Check sheet for the modelled part. Datum: model origin and axes. Units: mm. A direction names the side the tool comes from. Round coordinates to 2 decimals unless told otherwise and drop trailing zeros. Write each loop counter-clockwise with the first axis right and the second up, starting at its lowest first coordinate (ties: lowest second). Pieces come first, ordered by that corner, then holes. Notation, with made-up numbers: M -16,40.5 L -3,40.5 A19 ccw -3,50.5 Z; hole C 61,-30 d5. An arc over 180 degrees is marked long. Answer in a Markdown table with one row per item.
```python
from build123d import *

# Parameters (mm, degrees)
SKETCH1_W           = 550
SKETCH1_H           = 105
SKETCH1_R           = 50
BOSS_EXTRUDE2_DEPTH = 80
FILLET4_R           = 50
FILLET5_R           = 50
SKETCH11_W          = 150
SKETCH11_H          = 104.268109322
BOSS_EXTRUDE3_DEPTH = 80
SKETCH12_R          = 5
BOSS_EXTRUDE4_DEPTH = 120
FILLET8_R           = 50
FILLET9_R           = 50
FILLET10_R          = 50
SKETCH13_R          = 16.1
CUT_EXTRUDE1_DEPTH  = 150


with BuildPart() as part:
    # Sketch1 → Boss-Extrude2 (new body)
    with BuildSketch(Plane(origin=(0, 0, 0), x_dir=(1, 0, 0), z_dir=(0, 1, 0))):
        Rectangle(SKETCH1_W, SKETCH1_H)
        with Locations((-220, 0)):
            Circle(SKETCH1_R, mode=Mode.SUBTRACT)
        with Locations((125, 0)):
            Circle(SKETCH1_R, mode=Mode.SUBTRACT)
    extrude(amount=BOSS_EXTRUDE2_DEPTH)

    # Fillet4
    fillet4_edges = [part.edges().sort_by_distance(p)[0] for p in [
        (275, 40, 52.5),
    ]]
    fillet(fillet4_edges, radius=FILLET4_R)

    # Fillet5
    fillet5_edges = [part.edges().sort_by_distance(p)[0] for p in [
        (275, 40, -52.5),
    ]]
    fillet(fillet5_edges, radius=FILLET5_R)

    # Sketch11 → Boss-Extrude3 (add)
    with BuildSketch(Plane(origin=(0, 80, 0), x_dir=(1, 0, 0), z_dir=(0, 1, 0))):
        with Locations((-200, 0.365945339)):
            Rectangle(SKETCH11_W, SKETCH11_H)
    extrude(amount=BOSS_EXTRUDE3_DEPTH)

    # Sketch12 → Boss-Extrude4 (add)
    with BuildSketch(Plane.XZ.offset(-80)):
        with Locations((-220, 0)):
            Circle(SKETCH12_R)
    extrude(amount=BOSS_EXTRUDE4_DEPTH)

    # Fillet8
    fillet8_edges = [part.edges().sort_by_distance(p)[0] for p in [
        (-275, 40, 52.5),
    ]]
    fillet(fillet8_edges, radius=FILLET8_R)

    # Fillet9
    fillet9_edges = [part.edges().sort_by_distance(p)[0] for p in [
        (-275, 80, -52.5),
    ]]
    fillet(fillet9_edges, radius=FILLET9_R)

    # Fillet10
    fillet10_edges = [part.edges().sort_by_distance(p)[0] for p in [
        (-125, 160, -0.365945339),
    ]]
    fillet(fillet10_edges, radius=FILLET10_R)

    # Sketch13 → Cut-Extrude1 (cut)
    with BuildSketch(Plane(origin=(275, 0, 0), x_dir=(0, 0, -1), z_dir=(1, 0, 0))):
        with Locations((0, 23.9)):
            Circle(SKETCH13_R)
    extrude(amount=-CUT_EXTRUDE1_DEPTH, mode=Mode.SUBTRACT)


solid = part.part
```
1. Draft check along X on faces 1 (the face through (85, 39, 30)), 2 (the face through (-215.23, 20.84, 1.5)), 3 (the face through (-260.742, 78.88, -37.464)), 4 (the face through (-180, 119, 51.768)). Enter one of: +X half, -X half, draft (parallel to the pull), parting line (faces both ways), or undercut.
Found:
| item | result |
|---|---|
| face 1 | undercut |
| face 2 | undercut |
| face 3 | -X half |
| face 4 | draft |
2. Scan lines: L1, parallel to Y at x = 211, z = 0; L2, parallel to Z at x = 125, y = 33; L3, parallel to Z at x = -220, y = 23. Record each from-to range of solid material in increasing order.
Found:
| item | result |
|---|---|
| L1 | y = 0 to 7.8, 40 to 80 |
| L2 | z = -52.5 to -50, 50 to 52.5 |
| L3 | z = -52.5 to -50, -5 to 5, 50 to 52.5 |
3. Section check A-A, the plane x = 125. Record the cut outline in (y, z).
Found:
| item | result |
|---|---|
| outline | M 0,-52.5 L 80,-52.5 L 80,-50 L 0,-50 Z; M 0,50 L 80,50 L 80,52.5 L 0,52.5 Z |
4. Section check B-B, the plane z = 42. Record the cut outline in (x, y), and give its area (3 significant figures).
Found:
| item | result |
|---|---|
| outline | M -255.66,0 L -247.13,0 L -247.13,80 L -192.87,80 L -192.87,0 L 97.87,0 L 97.87,80 L -125,80 L -125,110 A50 ccw -175,160 L -255.66,160 Z; M 152.13,0 L 255.66,0 L 255.66,80 L 152.13,80 Z |
| area | 42,100 mm2 |
5. Access from +Z, -Z, +X, -X, +Y, -Y to the whole of each face (thin tool, end or side, straight path). Record for faces 5 (the face through (-269.95, 39.44, -2.2)), 6 (the face through (-125, 95, 0)), 7 (the face through (259.964, 40.56, 38.242)), 8 (the face through (224.387, 8.183, 3.49)).
Found:
| item | result |
|---|---|
| face 5 | -Y |
| face 6 | +Z, -Z, +X, +Y |
| face 7 | +Z, +X, +Y, -Y |
| face 8 | +X |
6. Section check D-D, the plane y = 23.9. Record the cut outline in (x, z).
Found:
| item | result |
|---|---|
| outline | M -275,-2.5 A50 ccw -225,-52.5 L 225,-52.5 A50 ccw 273.11,-16.1 L 172.34,-16.1 A50 cw long 172.34,16.1 L 273.11,16.1 A50 ccw 225,52.5 L -225,52.5 A50 ccw -275,2.5 Z; C -220,0 d10; hole C -220,0 d100 |
7. Section check C-C, the plane x = 187.5. Record the cut outline in (y, z), and give its area (3 significant figures).
Found:
| item | result |
|---|---|
| outline | M 0,-52.5 L 80,-52.5 L 80,52.5 L 0,52.5 Z; hole C 23.9,0 d32.2 |
| area | 7,590 mm2 |
8. Go/stop test with flat-tipped pins: pin 1 (4 mm diameter, centred on x = -140.5, z = -26.5, fed in from +Y); pin 2 (6 mm diameter, centred on y = 102, z = -18, fed in from +X); pin 3 (1 mm diameter, centred on y = 108, z = -19.5, fed in from -X). Record where each tip stops, or that it passes through.
Found:
| item | result |
|---|---|
| pin 1 | stops at y = 148 |
| pin 2 | stops at x = -125 |
| pin 3 | stops at x = -272.2 |
